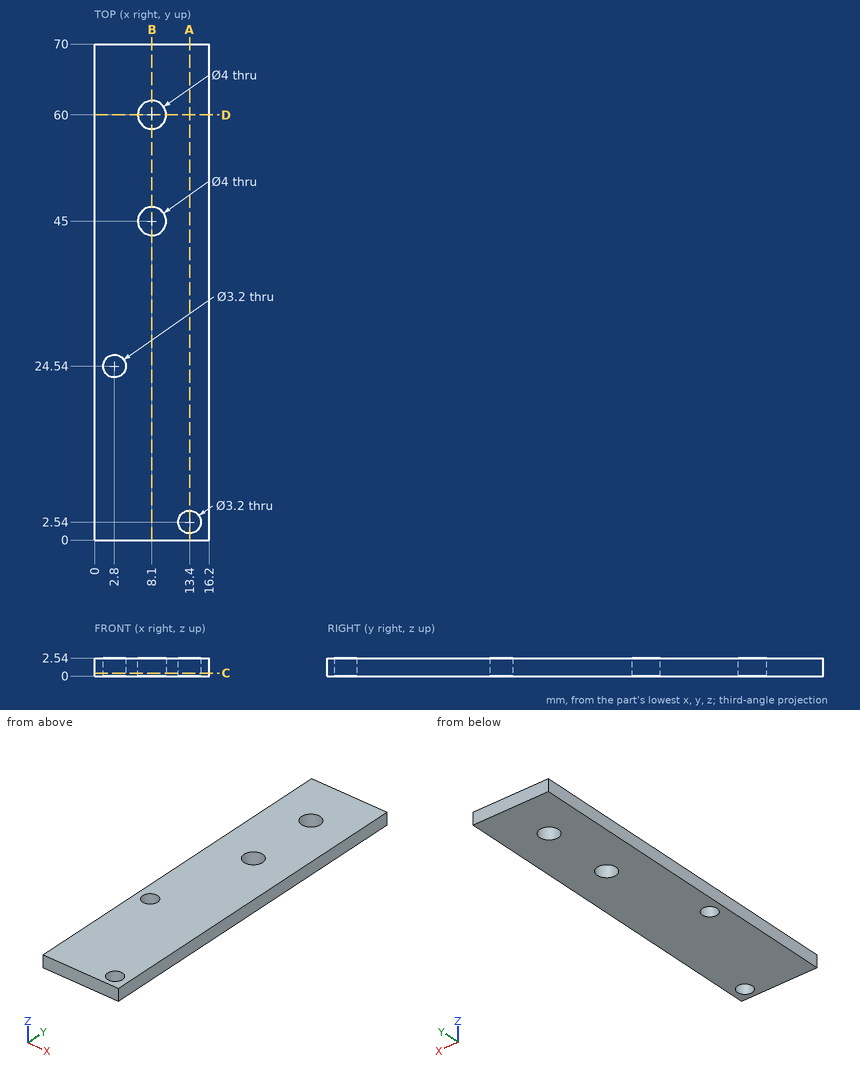
The drawing under review shows one solid part. Ordinate dimensions are in mm from its lowest x, y, z. Give positions to 0.01 mm unless a question says otherwise; leave off trailing zeros. Loops run counter-clockwise (first coordinate to the right, second up) from the corner with the lowest first, then second, coordinate; pieces in that order, holes last. Notation, with made-up numbers: M -39,12.25 L -27,12.25 A8 ccw -27,20.25 Z; hole C 44.25,-14.5 d9. An arc over 180 degrees is marked long. Return JSON: item names as keys, results as strings. Group by question number.
Item 1: We need section A-A (x = 13.4). Give the boundary of the cut face in (y, z).
Item 2: Insertion check: pin 1 Ø2.5 at (x, y) = (2.8, 24.54) entering from +Z. The pin has a flat end and moves straight along its axis. Give the tip position at first contact, or say it passes through.
Item 3: We need section B-B (x = 8.1). Give the boundary of the cut face in (y, z), and give its area (3 significant figures).
Item 4: We need section C-C (z = 0.4). Give the boundary of the cut face in (x, y).
Item 5: For probe 1 along Y at (x, z) = (8.1, 1.1); probe 2 along Y at (x, z) = (13.4, 1.75); probe 3 along Y at (x, z) = (7, 1), list the stretches that pass through material, from the lowest coordinate up.
Item 6: We need section D-D (y = 60). Give the boundary of the cut face in (x, z), and give its area (3 significant figures).
Output:
{
 "1": {"outline": "M 0,0 L 0.94,0 L 0.94,2.54 L 0,2.54 Z; M 4.14,0 L 70,0 L 70,2.54 L 4.14,2.54 Z"},
 "2": {"pin 1": "passes through"},
 "3": {"outline": "M 0,0 L 43,0 L 43,2.54 L 0,2.54 Z; M 47,0 L 58,0 L 58,2.54 L 47,2.54 Z; M 62,0 L 70,0 L 70,2.54 L 62,2.54 Z", "area": "157 mm^2"},
 "4": {"outline": "M 0,0 L 16.2,0 L 16.2,70 L 0,70 Z; hole C 2.8,24.54 d3.2; hole C 8.1,45 d4; hole C 8.1,60 d4; hole C 13.4,2.54 d3.2"},
 "5": {"probe 1": "y = 0 to 43, 47 to 58, 62 to 70", "probe 2": "y = 0 to 0.94, 4.14 to 70", "probe 3": "y = 0 to 43.33, 46.67 to 58.33, 61.67 to 70"},
 "6": {"outline": "M 0,0 L 6.1,0 L 6.1,2.54 L 0,2.54 Z; M 10.1,0 L 16.2,0 L 16.2,2.54 L 10.1,2.54 Z", "area": "31.0 mm^2"}
}
